The model under review builds one solid part; all positions refer to its coordinate system, in mm. Give positions to 0.01 mm unless a question says otherwise; leave off trailing zeros. Use CSV: the item, a comma, the result in double quotes.
```python
from build123d import *

# Parameters (mm, degrees)
BOSS_EXTRU_1_DEPTH   = 3
EMPREINTE1_OUTLINE_R = 1.938
EMPREINTE1_DEPTH     = 3


# Read off the part's stored shape, not the designer's step: Empreinte1
with BuildPart() as part:
    # Esquisse1 → Boss.-Extru.1 (new body)
    with BuildSketch(Plane.XY):
        with BuildLine():
            Line((2, 0), (28, 0))
            ThreePointArc((28, 0), (29.414213562, 0.585786438), (30, 2))
            Line((30, 2), (30, 118))
            ThreePointArc((30, 118), (29.414213562, 119.414213562), (28, 120))
            Line((28, 120), (2, 120))
            ThreePointArc((2, 120), (0.585786438, 119.414213562), (0, 118))
            Line((0, 118), (0, 2))
            ThreePointArc((0, 2), (0.585786438, 0.585786438), (2, 0))
        make_face()
    extrude(amount=BOSS_EXTRU_1_DEPTH)

    # Empreinte1 outline → Empreinte1 (cut)
    with BuildSketch(Plane.XY):
        with Locations((26.535185944, 116.535185944)):
            Circle(EMPREINTE1_OUTLINE_R)
        with Locations((3.460697179, 93.460697179)):
            Circle(EMPREINTE1_OUTLINE_R)
        with Locations((26.535185944, 86.535185944)):
            Circle(EMPREINTE1_OUTLINE_R)
        with Locations((3.460697179, 63.460697179)):
            Circle(EMPREINTE1_OUTLINE_R)
        with Locations((26.535185944, 56.535185944)):
            Circle(EMPREINTE1_OUTLINE_R)
        with Locations((3.460697179, 33.460697179)):
            Circle(EMPREINTE1_OUTLINE_R)
        with Locations((26.535185944, 26.535185944)):
            Circle(EMPREINTE1_OUTLINE_R)
        with Locations((3.460697179, 3.460697179)):
            Circle(EMPREINTE1_OUTLINE_R)
    extrude(amount=EMPREINTE1_DEPTH, mode=Mode.SUBTRACT)


solid = part.part
```
Item 1: Mouldability with a two-part tool opening along Y and no side actions: class faces 1 (the face through (3.208, 65.382, 1.479)), 2 (the face through (15, 0, 1)), 3 (the face through (15, 61, 3)) as pulls with the +Y half, pulls with the -Y half, needs draft (parallel to the pull), parting line crosses it, or undercut.
Results list:
face 1,"undercut"
face 2,"pulls with the -Y half"
face 3,"needs draft"
Item 2: Wall thickness on L1, parallel to Y at x = 26.5, z = 1.8; L2, parallel to Y at x = 25, z = 1.95; L3, parallel to X at y = 88, z = 0.85: over which ranges is each line inside the solid? List them lowest first.
Results list:
L1,"y = 0 to 24.6, 28.47 to 54.6, 58.47 to 84.6, 88.47 to 114.6, 118.47 to 120"
L2,"y = 0 to 25.35, 27.72 to 55.35, 57.72 to 85.35, 87.72 to 115.35, 117.72 to 120"
L3,"x = 0 to 25.27, 27.8 to 30"
Item 3: Take a section at A-A, the plane z = 1.9. State how many separate pieces and enclosed holes the cut face has, and give its area (3 significant figures).
Results list:
separate pieces,"1"
enclosed holes,"8"
area,"3,500 mm2"
